Can you work these out from the model? Positions are in its coordinate system, mm. A direction names the side the tool comes from. Round coordinates to 2 decimals unless told otherwise and drop trailing zeros. Order: outer loops, then holes, each group sorted by start corner. A loop starts at its lowest first (then second) coordinate and runs counter-clockwise, first axis right, second up.
from build123d import *

# Parameters (mm, degrees)
F0_W           = 80
F0_H           = 60
F0_R           = 12.5
F1_DEPTH       = 15
F3_D           = 7
F3_CBORE_D     = 11.25
F3_CBORE_DEPTH = 6
F4_R           = 5
F5_SIZE        = 1


with BuildPart() as f1:
    # F0 (on Front) → F1 (new body)
    with BuildSketch(Plane.XZ):
        Rectangle(F0_W, F0_H)
        Circle(F0_R, mode=Mode.SUBTRACT)
    extrude(amount=F1_DEPTH)

    # F3 (through all)
    with Locations(Plane.XZ.offset(15)):
        with Locations((-30, 20), (30, 20)):
            CounterBoreHole(F3_D / 2, F3_CBORE_D / 2, F3_CBORE_DEPTH)

    # F4
    f4_edges = [f1.edges().sort_by_distance(p)[0] for p in [
        (40, -7.5, 30),
        (40, -7.5, -30),
        (-40, -7.5, 30),
        (-40, -7.5, -30),
    ]]
    fillet(f4_edges, radius=F4_R)

    # F5
    f5_edges = [f1.edges().sort_by_distance(p)[0] for p in [
        (-12.5, -15, 0),
    ]]
    chamfer(f5_edges, length=F5_SIZE)


solid = f1.part
(1) I want a section at C-C, the plane z = 20. List the corners of the cut face in (x, y) for me (3 decimals).
(2) If we mould it in two halves opening along Z, with no side actions, what happens to faces 3 (the face through (-30.732, -12.042, 25.577)), 4 (the face through (-1, -15, 14)), 5 (the face through (38, -8, -29))? For each: pulls with the +Z half, pulls with the -Z half, needs draft (parallel to the pull), parting line crosses it, or undercut.
(3) I want a section at A-A, the plane z = 0. List the corners of the cut face in (x, y) for me.
(4) Please list where these lines run through material, in increasing order: probe 1 along Z at (x, y) = (30, -6); probe 2 along X at (y, z) = (-9.5, 15.5) (3 decimals); probe 3 along X at (y, z) = (-7.5, 19.5).
(5) I want a section at B-B, the plane x = -30. List the corners of the cut face in (y, z) for me (3 decimals), plus the area to 4 significant figures.
(6) I want a section at D-D, the plane y = -8. List the corners of the cut face in (x, z) for me, plus the area to 3 significant figures.
(7) On a 3-axis mill with a long thin cutter (end or side, diameter ignored), from which of +Z, -Z, +X, -X, +Y, -Y can I reach the whole of each face in a straight line? I mean faces 1 (the face through (-1, 0, -13)), 2 (the face through (29.268, -12.042, 25.577)). Say none if no direction works.
(8) I'm going to push flat-ended pins straight in: pin 1 Ø12 at (x, z) = (-6, -3.5) entering from -Y; pin 2 Ø3.5 at (x, z) = (28, 20) entering from -Y. Where does each tip first touch, or does it pass through?
Ans:
1. outline: (-40, -15) - (-35.625, -15) - (-35.625, -9) - (-33.5, -9) - (-33.5, 0) - (-40, 0) - close; (-26.5, -9) - (-24.375, -9) - (-24.375, -15) - (24.375, -15) - (24.375, -9) - (26.5, -9) - (26.5, 0) - (-26.5, 0) - close; (33.5, -9) - (35.625, -9) - (35.625, -15) - (40, -15) - (40, 0) - (33.5, 0) - close
2. face 3: undercut
2. face 4: needs draft
2. face 5: pulls with the -Z half
3. outline: (-40, -15) - (-13.5, -15) - (-12.5, -14) - (-12.5, 0) - (-40, 0) - close; (12.5, -14) - (13.5, -15) - (40, -15) - (40, 0) - (12.5, 0) - close
4. probe 1: z = -30 to 16.5, 23.5 to 30
4. probe 2: x = -40 to -33.375, -26.625 to 26.625, 33.375 to 40
4. probe 3: x = -40 to -33.46, -26.54 to 26.54, 33.46 to 40
5. outline: (-15, -30) - (0, -30) - (0, 16.5) - (-9, 16.5) - (-9, 14.375) - (-15, 14.375) - close; (-15, 25.625) - (-9, 25.625) - (-9, 23.5) - (0, 23.5) - (0, 30) - (-15, 30) - close
5. area: 769.5 mm2
6. outline: (-40, -25) arc R5 ccw to (-35, -30) - (35, -30) arc R5 ccw to (40, -25) - (40, 25) arc R5 ccw to (35, 30) - (-35, 30) arc R5 ccw to (-40, 25) - close; hole circle Ø7 at (-30, 20); hole circle Ø25 at (0, 0); hole circle Ø7 at (30, 20)
6. area: 4,210 mm2
7. face 1: +Z, -Z, +X, -X, +Y
7. face 2: -Y
8. pin 1: stops at y = -14.45
8. pin 2: stops at y = -9
